Work out the finished part from the listing and answer in its coordinate system (mm). Face numbers are marked on the shaded views. Round coordinates to 2 decimals unless told otherwise and drop trailing zeros. Write each loop counter-clockwise with the first axis right and the second up, starting at its lowest first coordinate (ties: lowest second). Pieces come first, ordered by that corner, then holes. Notation, with made-up numbers: M -35.5,60 L 16.5,60 A17 ccw 16.5,91 Z; hole C 77,-18 d7. An arc over 180 degrees is marked long. One line per item, written item: value. Start each with the question number.
Q1. Find section A-A (y = 7.25). Write down the section's boundary in (x, z), and give its area (3 significant figures).
Q2. Find section B-B (x = -24). Write down the section's boundary in (y, z), and give its area (3 significant figures).
Q3. The mould has two halves that part along X. Classify the marked faces 1, 2, 3 and 4: released by +X, released by -X, zero draft, split by the parting line, or undercut.
Q4. Given pin 1 Ø12 at (x, y) = (-10, -5) entering from +Z; pin 2 Ø5.5 at (x, y) = (-22.89, 6.58) entering from +Z, each flat-ended and moving along its own axis, determine where each tip first touches the part or whether it passes through.
Q5. Find section C-C (x = -6). Write down the section's boundary in (y, z), and give its area (3 significant figures).
Q6. Consider probe 1 along Y at (x, z) = (16, 1.75); probe 2 along Z at (x, y) = (-16.5, -7.5); probe 3 along Y at (x, z) = (-1, 1). Determine where each line is inside the solid, lowest interval first.
Q7. Find section D-D (y = -3). Write down the section's boundary in (x, z), and give its area (3 significant figures).
from build123d import *

# Parameters (mm, degrees)
F0_W     = 59.7732812166
F0_H     = 27.1696727723
F1_DEPTH = 2.5
F2_T     = -2
F3_DEPTH = 5
F4_R     = 2
F6_D     = 4.4


with BuildPart() as f1:
    # F0 (on Top) → F1 (new body, symmetric)
    with BuildSketch(Plane.XY):
        Rectangle(F0_W, F0_H)
    extrude(amount=F1_DEPTH, both=True)

    # F2
    f2_openings = [f1.faces().sort_by_distance(p)[0] for p in [
        (0, 0, 2.5),
    ]]
    offset(amount=F2_T, openings=f2_openings)

    # F3 (add): a face of the model
    f3_faces = [f1.faces().sort_by_distance(p)[0] for p in [
        (0, 0, -2.5),
    ]]
    extrude(f3_faces, amount=F3_DEPTH)

    # F4
    f4_edges = [f1.edges().sort_by_distance(p)[0] for p in [
        (0, 11.584836, -0.5),
        (0, -11.584836, -0.5),
        (27.886641, 0, -0.5),
        (-27.886641, 0, -0.5),
    ]]
    fillet(f4_edges, radius=F4_R)

    # F6 (through all)
    with Locations(Plane.XY):
        with Locations((-22.8866406083, 6.5848363861)):
            Hole(F6_D / 2)


solid = f1.part
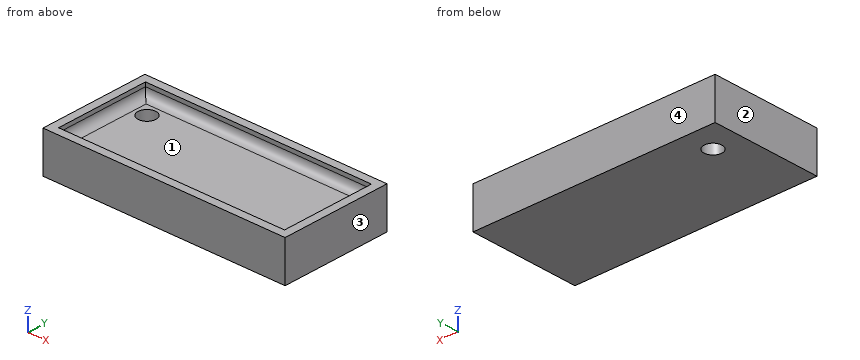
The answers:
1. outline: M -29.89,-7.5 L -24.98,-7.5 L -24.98,-0.5 L -25.89,-0.5 A2 cw -27.89,1.5 L -27.89,2.5 L -29.89,2.5 Z; M -20.79,-7.5 L 29.89,-7.5 L 29.89,2.5 L 27.89,2.5 L 27.89,1.5 A2 cw 25.89,-0.5 L -20.79,-0.5 Z
1. area: 403 mm2
2. outline: M -13.58,-7.5 L 4.69,-7.5 L 4.69,-0.5 L -9.58,-0.5 A2 cw -11.58,1.5 L -11.58,2.5 L -13.58,2.5 Z; M 8.48,-7.5 L 13.58,-7.5 L 13.58,2.5 L 11.58,2.5 L 11.58,1.5 A2 cw 9.58,-0.5 L 8.48,-0.5 Z
2. area: 177 mm2
3. face 1: undercut
3. face 2: released by -X
3. face 3: released by +X
3. face 4: zero draft
4. pin 1: z = 0.09
4. pin 2: z = -0.5
5. outline: M -13.58,-7.5 L 13.58,-7.5 L 13.58,2.5 L 11.58,2.5 L 11.58,1.5 A2 cw 9.58,-0.5 L -9.58,-0.5 A2 cw -11.58,1.5 L -11.58,2.5 L -13.58,2.5 Z
5. area: 204 mm2
6. probe 1: -13.58 to -11.58, 11.58 to 13.58
6. probe 2: -7.5 to -0.5
6. probe 3: -13.58 to -11.52, 11.52 to 13.58
7. outline: M -29.89,-7.5 L 29.89,-7.5 L 29.89,2.5 L 27.89,2.5 L 27.89,1.5 A2 cw 25.89,-0.5 L -25.89,-0.5 A2 cw -27.89,1.5 L -27.89,2.5 L -29.89,2.5 Z
7. area: 432 mm2
